Could you check a few things on this model? Use its own coordinates, in mm. A direction names the side the tool comes from. Round coordinates to 2 decimals unless told otherwise and drop trailing zeros. Write each loop counter-clockwise with the first axis right and the second up, starting at its lowest first coordinate (ties: lowest second). Pieces come first, ordered by that corner, then holes. Notation, with made-up numbers: M -3,-26.5 L 44,-26.5 A16 ccw 44,-3.5 Z; hole C 77,19.5 d4. An arc over 180 degrees is marked long. One line per item, written item: value. Start each with the question number.
(1) If I drill on L1, parallel to Z at x = -25.4, y = 7.75 (3 decimals); L2, parallel to Z at x = -26, y = 11; L3, parallel to X at y = 11.5, z = 5.5, over which ranges is the centre line in solid material (lowest first)?
(2) I want a section at A-A on x = 8. Please give me the cut outline in (y, z) (3 decimals), and give its area (3 significant figures).
(3) I want a section at B-B on y = 2.25. Count the separate pieces of the cut face and the enclosed holes in it, and give its area (3 significant figures).
(4) I want a section at D-D on x = 26. Please give me the cut outline in (y, z).
(5) Thinking about a two-plate mould opening in X: for faces 1 (the face through (1, 0, 4)), 2 (the face through (44.45, 6, 0)), 3 (the face through (57.15, 6.26, -0.14)), which applies, released by +X, released by -X, zero draft, split by the parting line, or undercut?
(6) Which directions (+Z, -Z, +X, -X, +Y, -Y) give clear straight access to the entire face, cutting with the end or side of a thin tool? Please do faces 4 (the face through (-31.75, 6, 0)), 5 (the face through (-1, 6, 6.35)).
(7) I'm going to push flat-ended pins straight in: pin 1 Ø1 at (y, z) = (2, -4.5) entering from -X; pin 2 Ø4 at (y, z) = (4, 3.5) entering from +X. Where does each tip first touch, or does it pass through?
Autodesk Inventor part; units mm, degrees
ref_plane "YZ Plane" through (0, 0, 0) normal (1, 0, 0) x (0, 1, 0)
ref_plane "XZ Plane" through (0, 0, 0) normal (0, 1, 0) x (-1, 0, 0)
ref_plane "XY Plane" through (0, 0, 0) normal (0, 0, 1) x (1, 0, 0)
sketch "Sketch1" plane through (0, 0, 0) normal (0, 1, 0) x (-1, 0, 0)
  line L0 (50.8, 6.35) -> (-50.8, 6.35)
  line L1 (-50.8, -6.35) -> (50.8, -6.35)
  arc A0 (50.8, -6.35) -> (50.8, 6.35) centre (50.8, 0) ccw
  arc A1 (-50.8, 6.35) -> (-50.8, -6.35) centre (-50.8, 0) ccw
  line L2 (80.01, 0) -> (-80.01, 0)
  line L3 (0, -8.89) -> (0, 8.89)
  point P0 (0, 0)
  dimension "d2" = 101.6
  dimension "d3" = 6.35
  dimension "d4" = 6.35
  dimension "d5" = 50.8
  dimension "d6" = 0
  dimension "d7" = 12.7
  dimension "d8" = 101.6
  dimension "d9" = 6.35
extrude "Extrusion1" add sketch "Sketch1" along normal blind 12.7
sketch "Sketch2" plane through (0, 12.7, 0) normal (0, 1, 0) x (1, 0, 0)
  circle A0 centre (-50.8, 0) radius 3.175
  line L0 (-80.01, 0) -> (80.01, 0)
  line L1 (0, 8.89) -> (0, -8.89)
  circle A1 centre (-25.4, 0) radius 3.175
  circle A2 centre (0, 0) radius 3.175
  circle A3 centre (25.4, 0) radius 3.175
  circle A4 centre (50.8, 0) radius 3.175
  dimension "d12" = 6.35
  dimension "d13" = 50.8
  dimension "d14" = 0
  dimension "d17" = 25.4
extrude "Extrusion2" cut sketch "Sketch2" against normal through all
sketch "Sketch3" plane through (0, 12.7, 0) normal (0, 1, 0) x (1, 0, 0)
  line L0 (-44.45, -3.175) -> (-31.75, -3.175)
  line L1 (-31.75, -3.175) -> (-31.75, 3.175)
  line L2 (-31.75, 3.175) -> (-44.45, 3.175)
  line L3 (-44.45, 3.175) -> (-44.45, -3.175)
  line L4 (-84.8983, 0) -> (80.8247, 0)
  line L5 (0, 12.3762) -> (0, -29.8073)
  line L6 (-6.35, 3.175) -> (-19.05, 3.175)
  line L7 (-6.35, -3.175) -> (-6.35, 3.175)
  line L8 (-19.05, 3.175) -> (-19.05, -3.175)
  line L9 (-19.05, -3.175) -> (-6.35, -3.175)
  line L10 (19.05, 3.175) -> (6.35, 3.175)
  line L11 (19.05, -3.175) -> (19.05, 3.175)
  line L12 (6.35, 3.175) -> (6.35, -3.175)
  line L13 (6.35, -3.175) -> (19.05, -3.175)
  line L14 (44.45, 3.175) -> (31.75, 3.175)
  line L15 (44.45, -3.175) -> (44.45, 3.175)
  line L16 (31.75, 3.175) -> (31.75, -3.175)
  line L17 (31.75, -3.175) -> (44.45, -3.175)
  point P0 (0, 0)
  dimension "d24" = 12.7
  dimension "d25" = 6.35
  dimension "d26" = 31.75
  dimension "d27" = 3.175
  dimension "d30" = 25.4
extrude "Extrusion3" cut sketch "Sketch3" against normal through all
properties part number "4M Module" material "Wood (Oak)"
Found:
1. L1: z = -6.35 to -3.175, 3.175 to 6.35
1. L2: z = -6.35 to -3.12, 3.12 to 6.35
1. L3: x = -53.97 to 53.97
2. outline: M 0,-6.35 L 12.7,-6.35 L 12.7,-3.175 L 0,-3.175 Z; M 0,3.175 L 12.7,3.175 L 12.7,6.35 L 0,6.35 Z
2. area: 80.6 mm²
3. separate pieces: 1
3. enclosed holes: 9
3. area: 936 mm²
4. outline: M 0,-6.35 L 12.7,-6.35 L 12.7,-3.12 L 0,-3.12 Z; M 0,3.12 L 12.7,3.12 L 12.7,6.35 L 0,6.35 Z
5. face 1: zero draft
5. face 2: undercut
5. face 3: released by +X
6. face 4: +Y, -Y
6. face 5: +Z, +X, -X, +Y, -Y
7. pin 1: stops at x = -55.73
7. pin 2: stops at x = 56.97
